```python
from build123d import *

# Parameters (mm, degrees)
SKETCH2_R                        = 3
BOSS_EXTRUDE1_DEPTH              = 1
SKETCH3_R                        = 2.5
BOSS_EXTRUDE2_DEPTH              = 1.6
SKETCH4_R                        = 1.5
BOSS_EXTRUDE3_DEPTH              = 9.15
CUT_EXTRUDE1_DEPTH               = 7.8
DRAFT1_ANGLE                     = 44.5
F_14_5_14_5_DIAMETER_HOLE1_D     = 14.5
F_14_5_14_5_DIAMETER_HOLE1_DEPTH = 2.35
F_1_6_1_6_DIAMETER_HOLE1_D       = 1.6
F_1_6_1_6_DIAMETER_HOLE1_DEPTH   = 3
F_1_6_1_6_DIAMETER_HOLE1_TIP     = 0.480688495


with BuildPart() as part:
    # Sketch1 → Revolve1 (revolve)
    with BuildSketch(Plane.XY):
        with BuildLine():
            Line((0, 8), (0, 0))
            Line((0, 0), (15.15, 0))
            Line((15.15, 0), (15.15, 8))
            Line((15.15, 8), (2.05, 8))
            ThreePointArc((2.05, 8), (2, 7.98660254), (1.95, 8))
            Line((1.95, 8), (0, 8))
        make_face()
    revolve(axis=Axis((0, 0, 0), (1, 0, 0)))

    # Sketch2 → Boss-Extrude1 (add)
    with BuildSketch(Plane.ZY):
        Circle(SKETCH2_R)
    extrude(amount=BOSS_EXTRUDE1_DEPTH)

    # Sketch3 → Boss-Extrude2 (add)
    with BuildSketch(Plane.ZY.offset(1)):
        Circle(SKETCH3_R)
    extrude(amount=BOSS_EXTRUDE2_DEPTH)

    # Sketch4 → Boss-Extrude3 (add)
    with BuildSketch(Plane.ZY.offset(2.6)):
        Circle(SKETCH4_R)
    extrude(amount=BOSS_EXTRUDE3_DEPTH)

    # Sketch5 → Cut-Extrude1 (cut)
    with BuildSketch(Plane.ZY.offset(11.75)):
        with BuildLine():
            Line((-0.748331477, 1.3), (0.748331477, 1.3))
            ThreePointArc((0.748331477, 1.3), (0, 1.5), (-0.748331477, 1.3))
        make_face()
    extrude(amount=-CUT_EXTRUDE1_DEPTH, mode=Mode.SUBTRACT)

    # Draft1
    draft1_faces = [part.faces().sort_by_distance(p)[0] for p in [
        (-3.95, 1.380475515, 0),
    ]]
    draft(draft1_faces, Plane(origin=(-3.95, 1.3, -0.748331477), x_dir=(0, 0, 1), z_dir=(0, 1, 0)), DRAFT1_ANGLE)

    # Ø14.5 (14.5) Diameter Hole1
    with Locations(Plane(origin=(15.15, 0, 0), x_dir=(0, 0, -1), z_dir=(1, 0, 0))):
        with Locations((0, 0)):
            Hole(F_14_5_14_5_DIAMETER_HOLE1_D / 2, depth=F_14_5_14_5_DIAMETER_HOLE1_DEPTH)

    # Ø1.6 (1.6) Diameter Hole1
    with Locations(Plane.ZY):
        with Locations((8.727e-06, 5), (4.330131382, 2.499992442), (4.330122656, -2.500007557), (-8.727e-06, -5), (-4.330131382, -2.499992442), (-4.330122656, 2.500007557)):
            Hole(F_1_6_1_6_DIAMETER_HOLE1_D / 2, depth=F_1_6_1_6_DIAMETER_HOLE1_DEPTH)
            with Locations((0, 0, -(F_1_6_1_6_DIAMETER_HOLE1_DEPTH + F_1_6_1_6_DIAMETER_HOLE1_TIP / 2))):  # 118° drill point
                Cone(0, F_1_6_1_6_DIAMETER_HOLE1_D / 2, F_1_6_1_6_DIAMETER_HOLE1_TIP, mode=Mode.SUBTRACT)


solid = part.part
```
Geometry check sheet. Reference: the model listing, model coordinates, mm. A direction names the side the tool comes from. Round coordinates to 2 decimals unless told otherwise and drop trailing zeros. Order: outer loops, then holes, each group sorted by start corner. A loop starts at its lowest first (then second) coordinate and runs counter-clockwise, first axis right, second up. Notation, with made-up numbers: (10, 36) - (35, 36) arc R11 ccw to (35, 54) - close; hole circle Ø7 at (86, -4.5). An arc over 180 degrees is marked (long way). Use a Markdown table: item, result. Add a question column.
1) Thickness scan on line 1 along X through (y, z) = (-6.75, -1.5); line 2 along Z through (x, y) = (0.75, 5) (3 decimals); line 3 along Y through (x, z) = (0.25, -5.75). Record the ranges inside material, lowest first.
2) Set-up check for faces 1 (the flat face through (-11.75, 0, 0)), 2 (the cylindrical face through (1.52, 2.01, 4.96)), 3 (the flat face through (12.8, 0, 0)): record each of +Z, -Z, +X, -X, +Y, -Y from which the full face is reachable in a straight line by a thin tool's end or side.
3) Section check A-A (y = 0). Record the cut outline in (x, z).
4) Section check C-C (x = 12.25). Record the cut outline in (y, z).
5) Mould release check, pull along Z, two halves, no side actions. Record for faces 4 (the cylindrical face through (1.52, 4.22, 0.17)), 5 (the flat face through (-1, 2, -2)), 6 (the cylindrical face through (8.51, -1.73, -7.81)): released by +Z, released by -Z, zero draft, split by the parting line, or undercut.
6) Section check B-B (x = -4.5). Record the cut outline in (y, z), then the cut area to 3 significant figures.
7) Gauge pin test, flat ends, axial feed: P1, Ø7, axis at y = 0, z = -0.5, coming from the +X side; P2, Ø1.8, axis at y = -5, z = 0, coming from the -X side; P3, Ø4, axis at x = -6, y = 3.5, coming from the +Z side; P4, Ø1.2, axis at x = -8, z = 0, coming from the +Y side. Record the tip position at first contact, or that the pin passes through.
Established:
| question | item | result |
|---|---|---|
| 1 | line 1 | 0 to 12.8 |
| 1 | line 2 | -6.245 to -0.8, 0.8 to 6.245 |
| 1 | line 3 | -5.56 to 5.56 |
| 2 | face 1 | +Z, -Z, -X, +Y, -Y |
| 2 | face 2 | -X |
| 2 | face 3 | +X |
| 3 | outline | (-11.75, -1.5) - (-2.6, -1.5) - (-2.6, -2.5) - (-1, -2.5) - (-1, -3) - (0, -3) - (0, -8) - (1.95, -8) arc R0.1 cw to (2.05, -8) - (15.15, -8) - (15.15, -7.25) - (12.8, -7.25) - (12.8, 7.25) - (15.15, 7.25) - (15.15, 8) - (2.05, 8) arc R0.1 cw to (1.95, 8) - (0, 8) - (0, 3) - (-1, 3) - (-1, 2.5) - (-2.6, 2.5) - (-2.6, 1.5) - (-11.75, 1.5) - close |
| 4 | outline | circle Ø16 at (0, 0) |
| 5 | face 4 | undercut |
| 5 | face 5 | zero draft |
| 5 | face 6 | split by the parting line |
| 6 | outline | (1.3, -0.75) - (1.3, 0.75) arc R1.5 ccw (long way) to start |
| 6 | area | 6.87 mm2 |
| 7 | P1 | x = 12.8 |
| 7 | P2 | x = 0 |
| 7 | P3 | through |
| 7 | P4 | y = 1.3 |
